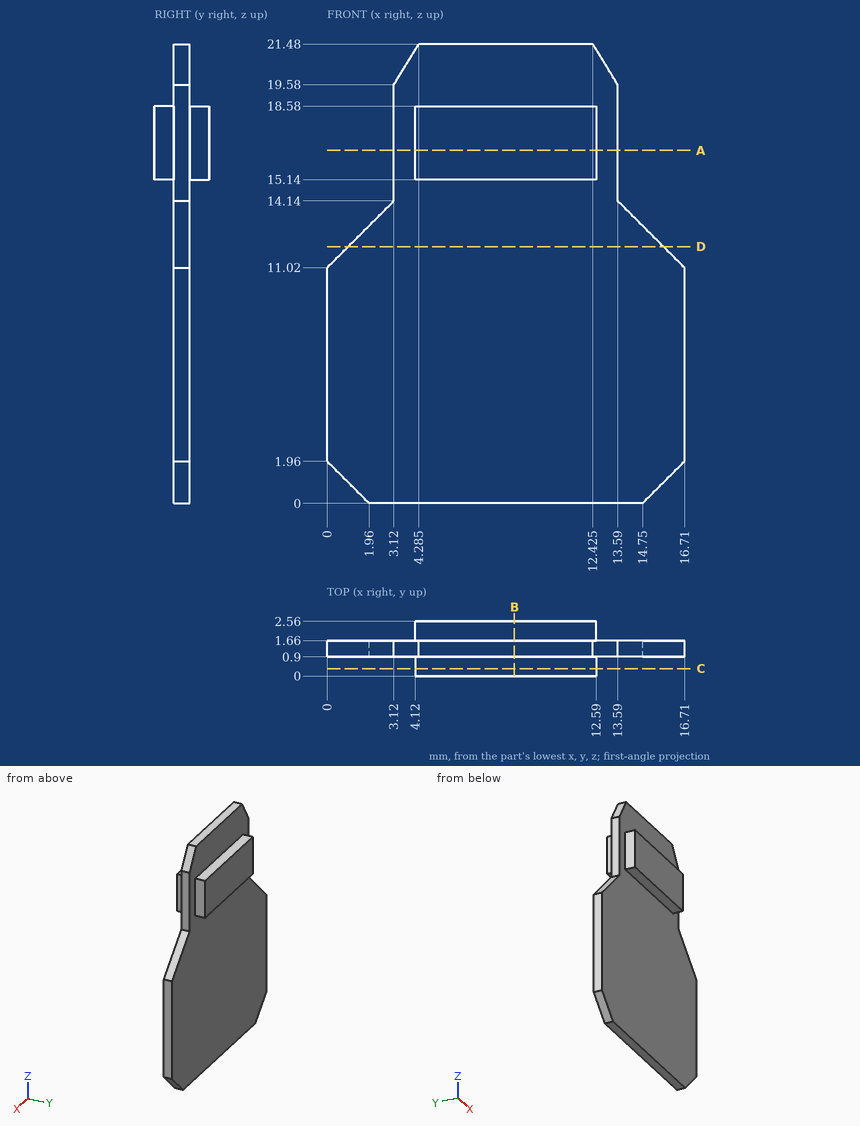
Answer from the drawing. Dimensions are ordinates in mm from the lowest x, y and z of the part. Give positions to 0.01 mm unless a question says otherwise; leave off trailing zeros. Write each loop counter-clockwise with the first axis right and the second up, starting at its lowest first coordinate (ties: lowest second). Pieces come first, ordered by that corner, then holes.
1) Section D-D (z = 12) is taken. Write down the section's boundary in (x, y).
2) Find the intervals of material crossed by L1, parallel to Z at x = 7.5, y = 1.9; L2, parallel to Y at x = 7.5, z = 6.5; L3, parallel to Z at x = 4, y = 0.95, in increasing order.
3) Section B-B (x = 8.75) is taken. Write down the section's boundary in (y, z).
4) Section A-A (z = 16.5) is taken. Write down the section's boundary in (x, y).
5) Given P1, Ø3, axis at x = 14, z = 11.5, coming from the -Y side; P2, Ø4, axis at x = 15, z = 13.5, coming from the +Y side; P3, Ø5, axis at x = 11, z = 13, coming from the -Y side; P4, Ø0.6, axis at y = 1.5, z = 18, coming from the +X side, each flat-ended and moving along its own axis, determine where each tip first touches the part or whether it passes through.
6) Section C-C (y = 0.35) is taken. Write down the section's boundary in (x, z).
Response:
1. outline: (0.98, 0.9) - (15.73, 0.9) - (15.73, 1.66) - (0.98, 1.66) - close
2. L1: z = 15.14 to 18.58
2. L2: y = 0.9 to 1.66
2. L3: z = 0 to 21.02
3. outline: (0, 15.14) - (0.9, 15.14) - (0.9, 0) - (1.66, 0) - (1.66, 15.14) - (2.56, 15.14) - (2.56, 18.58) - (1.66, 18.58) - (1.66, 21.48) - (0.9, 21.48) - (0.9, 18.58) - (0, 18.58) - close
4. outline: (3.12, 0.9) - (4.12, 0.9) - (4.12, 0) - (12.59, 0) - (12.59, 0.9) - (13.59, 0.9) - (13.59, 1.66) - (12.59, 1.66) - (12.59, 2.56) - (4.12, 2.56) - (4.12, 1.66) - (3.12, 1.66) - close
5. P1: stops at y = 0.9
5. P2: stops at y = 1.66
5. P3: stops at y = 0
5. P4: stops at x = 13.59
6. outline: (4.12, 15.14) - (12.59, 15.14) - (12.59, 18.58) - (4.12, 18.58) - close
